Solid Edge part; units mm, degrees
sketch "Sketch1" plane through (0, 0, 0) normal (0, -1, 0) x (1, 0, 0)
  line L0 (-7.9, 0) -> (7.9, 0)
  line L1 (7.9, 0) -> (7.9, 6.4)
  line L2 (7.9, 6.4) -> (16, 6.4)
  line L3 (16, 6.4) -> (16, 4.7)
  line L4 (7.9, -3.2) -> (16, 4.7)
  line L5 (-7.9, -3.2) -> (7.9, -3.2)
  line L6 (-7.9, -3.2) -> (-16, 4.7)
  line L7 (-16, 6.4) -> (-16, 4.7)
  line L8 (-7.9, 6.4) -> (-16, 6.4)
  line L9 (-7.9, 0) -> (-7.9, 6.4)
extrude "Protrusion1" add sketch "Sketch1" against normal blind 8
sketch "Sketch2" plane through (11.95, 4, 6.4) normal (0, 0, 1) x (1, 0, 0)
  line L0 (-2.7, -2.7) -> (2.7, -2.7)
  line L1 (2.7, -2.7) -> (2.7, 2.7)
  line L2 (2.7, 2.7) -> (-2.7, 2.7)
  line L3 (-2.7, 2.7) -> (-2.7, -2.7)
extrude "ExtrudedCutout_1" cut sketch "Sketch2" against normal blind 1.2
sketch "Sketch3" plane through (0, 4, 0) normal (0, 0, 1) x (1, 0, 0)
  circle A0 centre (-4, 0) radius 2.4
  circle A1 centre (4, 0) radius 2.4
extrude "ExtrudedProtrusion_2" add sketch "Sketch3" along normal blind 1.8
sketch "Sketch4" plane through (11.95, 4, 5.2) normal (0, 0, 1) x (1, 0, 0)
  circle A0 centre (0, 0) radius 2.4
  circle A1 centre (0, 0) radius 1.7
extrude "ExtrudedProtrusion_3" add sketch "Sketch4" along normal blind 3
mirror "Mirror1" about plane through (0, 0, 0) normal (1, 0, 0) of "ExtrudedCutout_1"
mirror "Mirror2" about plane through (0, 0, 0) normal (1, 0, 0) of "ExtrudedProtrusion_3"
sketch "Sketch5" plane through (0, 4, -3.2) normal (0, 0, -1) x (1, 0, 0)
  line L0 (-6.505, -2.5) -> (6.505, -2.5)
  line L1 (6.505, -2.5) -> (6.505, 2.5)
  line L2 (6.505, 2.5) -> (-6.505, 2.5)
  line L3 (-6.505, 2.5) -> (-6.505, -2.5)
  circle A0 centre (0, 0) radius 1.4
extrude "ExtrudedCutout_3" cut sketch "Sketch5" against normal blind 2
sketch "Sketch6" plane through (0, 4, -1.2) normal (0, 0, -1) x (1, 0, 0)
  circle A0 centre (-4, 0) radius 2.4
  circle A1 centre (4, 0) radius 2.4
extrude "ExtrudedCutout_4" cut sketch "Sketch6" against normal blind 0.0255
Verification items for the finished model (mm, model axes). A direction names the side the tool comes from. Coordinates: 2 decimals unless noted, no trailing zeros. Write each loop counter-clockwise with the first axis right and the second up, starting at its lowest first coordinate (ties: lowest second). Pieces come first, ordered by that corner, then holes. Notation, with made-up numbers: (-22.75, 77.5) - (-8.75, 77.5) arc R29 ccw to (-8.75, 99.5) - close; hole circle Ø10 at (87, 62.5). An arc over 180 degrees is marked (long way). Answer as a JSON object with one key per item and string values.
(1) Cross-section at A-A on x = 0. Record the cut outline in (y, z).
Report:
{"outline": "(0, -3.2) - (1.5, -3.2) - (1.5, -1.2) - (2.6, -1.2) - (2.6, -3.2) - (5.4, -3.2) - (5.4, -1.2) - (6.5, -1.2) - (6.5, -3.2) - (8, -3.2) - (8, 0) - (0, 0) - close"}
(2) Thickness scan on line 1 along Y through (x, z) = (11.95, 5.9); line 2 along Y through (x, z) = (11.95, 7.05); line 3 along Z through (x, y) = (-5, 3.5). Record the ranges inside material, lowest first.
Report:
{"line 1": "0 to 1.3, 1.6 to 2.3, 5.7 to 6.4, 6.7 to 8", "line 2": "1.6 to 2.3, 5.7 to 6.4", "line 3": "-1.17 to 1.8"}
(3) Cross-section at C-C on x = -11.95. Record the cut outline in (y, z), plus the area to 3 significant figures.
Report:
{"outline": "(0, 0.75) - (8, 0.75) - (8, 6.4) - (6.7, 6.4) - (6.7, 5.2) - (6.4, 5.2) - (6.4, 8.2) - (5.7, 8.2) - (5.7, 5.2) - (2.3, 5.2) - (2.3, 8.2) - (1.6, 8.2) - (1.6, 5.2) - (1.3, 5.2) - (1.3, 6.4) - (0, 6.4) - close", "area": "42.9 mm^2"}
(4) Mould release check, pull along X, two halves, no side actions. Record for faces 1 (the flat face through (0, 0, -1)), 2 (the flat face through (-11.9, 3.9, 0.7)), 3 (the flat face through (-7.9, 4, 3)): pulls with the +X half, pulls with the -X half, needs draft (parallel to the pull), parting line crosses it, or undercut.
Report:
{"face 1": "needs draft", "face 2": "pulls with the -X half", "face 3": "undercut"}
(5) Cross-section at D-D on z = -0.5. Record the cut outline in (x, y).
Report:
{"outline": "(-10.67, 0) - (10.67, 0) - (10.67, 8) - (-10.67, 8) - close"}
(6) Cross-section at B-B on z = 2.75. Record the cut outline in (x, y).
Report:
{"outline": "(-14, 0) - (-7.9, 0) - (-7.9, 8) - (-14, 8) - close; (7.9, 0) - (14, 0) - (14, 8) - (7.9, 8) - close"}
(7) Gauge pin test, flat ends, axial feed: pin 1 Ø4.5 at (x, y) = (-4, 4) entering from -Z; pin 2 Ø2 at (x, z) = (5, 4.5) entering from +Y; pin 3 Ø1 at (x, y) = (12.5, 4) entering from +Z; pin 4 Ø1.6 at (y, z) = (3, -2) entering from -X. Record the tip position at first contact, or that the pin passes through.
Report:
{"pin 1": "z = -1.17", "pin 2": "through", "pin 3": "z = 5.2", "pin 4": "x = -9.95"}
(8) Tool access check on faces 4 (the flat face through (-4, 4, -1.174)), 5 (the flat face through (-12, 1.3, 6)), 6 (the flat face through (-4, 4, 1.8)). Record the directions out of +Z, -Z, +X, -X, +Y, -Y that give a thin tool (end or side, any length) a straight path to the whole face; none if there is none.
Report:
{"face 4": "-Z", "face 5": "+Z", "face 6": "+Z, +Y, -Y"}
